Build history of the part. All positions in model axes, mm. Face numbers are marked on the shaded views. Give positions to 0.01 mm unless a question says otherwise; leave off trailing zeros. Write each loop counter-clockwise with the first axis right and the second up, starting at its lowest first coordinate (ties: lowest second). Pieces come first, ordered by that corner, then holes. Notation, with made-up numbers: (30.5, -10) -> (73.5, -10) arc R30 cw to (73.5, 21) -> close; hole circle Ø1 at (-25, 64.25). An arc over 180 degrees is marked (long way). Put each result on its own line as item: value.
from build123d import *

# Parameters (mm, degrees)
SKETCH1_R           = 35
BOSS_EXTRUDE1_DEPTH = 5
SKETCH2_R           = 2.25
CUT_EXTRUDE1_DEPTH  = 5
CIRPATTERN2_COUNT   = 4
SKETCH3_R           = 1.65
CUT_EXTRUDE2_DEPTH  = 5
CIRPATTERN3_COUNT   = 4
SKETCH4_R           = 7.5
CUT_EXTRUDE3_DEPTH  = 50.749371855


with BuildPart() as part:
    # Sketch1 → Boss-Extrude1 (new body)
    with BuildSketch(Plane(origin=(0, 0, 0), x_dir=(1, 0, 0), z_dir=(0, 1, 0))):
        with Locations(Location((0, 0, 0), (0, 0, 270))):
            Circle(SKETCH1_R)
    extrude(amount=BOSS_EXTRUDE1_DEPTH)

    # Sketch2 → Cut-Extrude1 (cut)
    with BuildSketch(Plane(origin=(0, 5, 0), x_dir=(1, 0, 0), z_dir=(0, 1, 0))):
        with Locations(Location((0, 28.285, 0), (0, 0, 270))):
            Circle(SKETCH2_R)
    cut_extrude1 = extrude(amount=-CUT_EXTRUDE1_DEPTH, mode=Mode.SUBTRACT)

    # CirPattern2: Cut-Extrude1 ×4 about axis
    cirpattern2_axis = Axis((0, 0, 0), (0, 1, 0))
    for i in range(1, CIRPATTERN2_COUNT):
        add(cut_extrude1.rotate(cirpattern2_axis, i * 360 / CIRPATTERN2_COUNT), mode=Mode.SUBTRACT)

    # Sketch3 → Cut-Extrude2 (cut)
    with BuildSketch(Plane(origin=(0, 5, 0), x_dir=(1, 0, 0), z_dir=(0, 1, 0))):
        with Locations(Location((0, 15, 0), (0, 0, 270))):
            Circle(SKETCH3_R)
    cut_extrude2 = extrude(amount=-CUT_EXTRUDE2_DEPTH, mode=Mode.SUBTRACT)

    # CirPattern3: Cut-Extrude2 ×4 about axis
    cirpattern3_axis = Axis((0, 0, 0), (0, 1, 0))
    for i in range(1, CIRPATTERN3_COUNT):
        add(cut_extrude2.rotate(cirpattern3_axis, i * 360 / CIRPATTERN3_COUNT), mode=Mode.SUBTRACT)

    # Sketch4 → Cut-Extrude3 (cut, through all)
    with BuildSketch(Plane(origin=(0, 5, 0), x_dir=(1, 0, 0), z_dir=(0, 1, 0))):
        with Locations(Location((0, 0, 0), (0, 0, 270))):
            Circle(SKETCH4_R)
    extrude(amount=-CUT_EXTRUDE3_DEPTH, mode=Mode.SUBTRACT)


solid = part.part
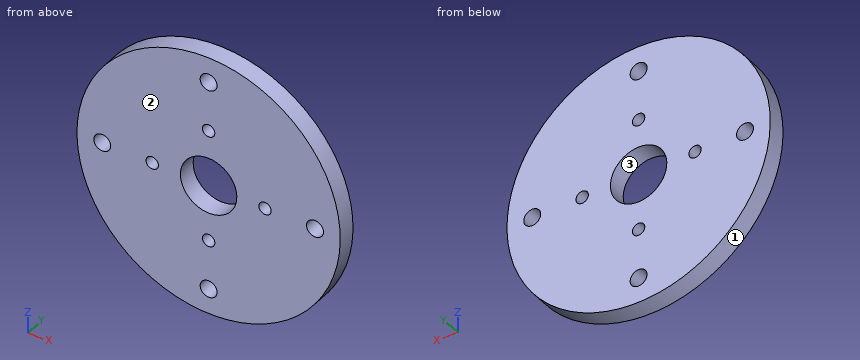
1) Slice it at D-D (z = -28). Write the cut outline in (x, y), plus the area to 3 significant figures.
Filled sheet:
outline: (-21, 0) -> (-2.23, 0) -> (-2.23, 5) -> (-21, 5) -> close; (2.23, 0) -> (21, 0) -> (21, 5) -> (2.23, 5) -> close
area: 188 mm2
2) Slice it at C-C (y = 2.7). Give the number of separate pieces and of enclosed holes in the cut face, plus the area to 3 significant figures.
Filled sheet:
separate pieces: 1
enclosed holes: 9
area: 3,570 mm2
3) Slice it at A-A (z = 0). Write the cut outline in (x, y) (3 decimals), plus the area to 3 significant figures.
Filled sheet:
outline: (-35, 0) -> (-30.535, 0) -> (-30.535, 5) -> (-35, 5) -> close; (-26.035, 0) -> (-16.65, 0) -> (-16.65, 5) -> (-26.035, 5) -> close; (-13.35, 0) -> (-7.5, 0) -> (-7.5, 5) -> (-13.35, 5) -> close; (7.5, 0) -> (13.35, 0) -> (13.35, 5) -> (7.5, 5) -> close; (16.65, 0) -> (26.035, 0) -> (26.035, 5) -> (16.65, 5) -> close; (30.535, 0) -> (35, 0) -> (35, 5) -> (30.535, 5) -> close
area: 197 mm2
4) Pin check, flat tips, straight feed: pin 1 (1.5 mm diameter, centred on x = -13.5, y = 4, fed in from +Z); pin 2 (1 mm diameter, centred on y = 3, z = 18.5, fed in from +X). Stop position of each tip, or through.
Filled sheet:
pin 1: z = 32.6
pin 2: x = 30.02
5) Wall check: L1, parallel to X at y = 3.4, z = -0.5; L2, parallel to X at y = 2.1, z = 16.5; L3, parallel to X at y = 2.8, z = 15. Give the ranges that are in metal, low to high.
Filled sheet:
L1: -35 to -30.48, -26.09 to -16.57, -13.43 to -7.48, 7.48 to 13.43, 16.57 to 26.09, 30.48 to 35
L2: -30.87 to -0.69, 0.69 to 30.87
L3: -31.62 to -1.65, 1.65 to 31.62
6) Pull direction Z, two halves, no side cores. Call the marked faces 1, 2 and 3: released by +Z, released by -Z, zero draft, split by the parting line, or undercut.
Filled sheet:
face 1: split by the parting line
face 2: zero draft
face 3: undercut
7) Slice it at B-B (x = 0). Write the cut outline in (y, z) (3 decimals), plus the area to 3 significant figures.
Filled sheet:
outline: (0, -35) -> (5, -35) -> (5, -30.535) -> (0, -30.535) -> close; (0, -26.035) -> (5, -26.035) -> (5, -16.65) -> (0, -16.65) -> close; (0, -13.35) -> (5, -13.35) -> (5, -7.5) -> (0, -7.5) -> close; (0, 7.5) -> (5, 7.5) -> (5, 13.35) -> (0, 13.35) -> close; (0, 16.65) -> (5, 16.65) -> (5, 26.035) -> (0, 26.035) -> close; (0, 30.535) -> (5, 30.535) -> (5, 35) -> (0, 35) -> close
area: 197 mm2
